Autodesk Inventor part; units mm, degrees
ref_plane "YZ Plane" through (0, 0, 0) normal (1, 0, 0) x (0, 1, 0)
ref_plane "XZ Plane" through (0, 0, 0) normal (0, 1, 0) x (-1, 0, 0)
ref_plane "XY Plane" through (0, 0, 0) normal (0, 0, 1) x (1, 0, 0)
sketch "Sketch1" plane through (0, 0, 0) normal (0, 0, 1) x (1, 0, 0)
  circle A0 centre (0, 0) radius 6.35
  dimension "d0" = 12.7
extrude "Extrusion1" add sketch "Sketch1" along normal blind 203.2
sketch "Sketch4" plane through (0, 0, 0) normal (0, 1, 0) x (-1, 0, 0)
  line L0 (0, 0) -> (0, 1.524)
  line L1 (6.35, 203.2) -> (-6.35, 203.2)
  line L2 (0, 203.2) -> (0, 201.676)
  circle A0 centre (0, 201.676) radius 1.27
  circle A1 centre (0, 1.524) radius 1.27
  dimension "d13" = 1.524
  dimension "d15" = 1.524
  dimension "d16" = 2.54
  dimension "d19" = 2.54
extrude "Extrusion4" cut sketch "Sketch4" along normal mid plane 15.24
sketch "Sketch5" plane through (0, 0, 0) normal (0, 1, 0) x (-1, 0, 0)
  line L0 (0, 1.524) -> (-1.27, 1.524)
  line L1 (-6.35, 0) -> (6.35, 0)
  line L2 (-1.27, 0) -> (1.27, 0)
  line L3 (1.27, 1.524) -> (0, 1.524)
  line L4 (1.27, 1.524) -> (6.35, 1.524)
  line L5 (6.35, 0) -> (6.35, 203.2)
  line L6 (6.35, 1.524) -> (-6.35, 1.524)
  line L7 (-6.35, 1.524) -> (-6.35, 0)
  line L8 (-6.35, 0) -> (6.35, 0)
  line L9 (6.35, 0) -> (6.35, 1.524)
  line L10 (6.35, 203.2) -> (-6.35, 203.2)
  line L11 (-6.35, 203.2) -> (6.35, 203.2)
  line L12 (6.35, 203.2) -> (6.35, 201.676)
  line L13 (6.35, 201.676) -> (-6.35, 201.676)
  line L14 (-6.35, 201.676) -> (-6.35, 203.2)
  point P0 (0, 0)
  dimension "d20" = 1.524
  dimension "d21" = 1.27
  dimension "d26" = 12.7
  dimension "d27" = 1.524
extrude "Extrusion6" cut sketch "Sketch5" along normal mid plane 25.4
sketch "Sketch7" plane through (0, 0, 0) normal (1, 0, 0) x (0, 1, 0)
  line L0 (0, 0) -> (0, 50.8)
  circle A0 centre (0, 50.8) radius 1.27
  line L1 (0, 50.8) -> (0, 101.6)
  circle A1 centre (0, 101.6) radius 1.27
  line L2 (0, 101.6) -> (0, 152.4)
  circle A2 centre (0, 152.4) radius 1.27
  dimension "d42" = 50.8
  dimension "d43" = 2.54
  dimension "d44" = 50.8
  dimension "d45" = 2.54
  dimension "d46" = 50.8
  dimension "d47" = 2.54
extrude "Extrusion8" cut sketch "Sketch7" along normal mid plane 25.4
properties part number "Straw"
Can you work these out from the model? Positions are in its coordinate system, mm. Give positions to 0.01 mm unless a question says otherwise; leave off trailing zeros. Write each loop counter-clockwise with the first axis right and the second up, starting at its lowest first coordinate (ties: lowest second). Pieces come first, ordered by that corner, then holes. Notation, with made-up numbers: (77, 59.5) -> (97, 59.5) arc R16 ccw to (97, 74.5) -> close; hole circle Ø6 at (31, 3). An arc over 180 degrees is marked (long way). One line per item, written item: value.
Q1. For P1, Ø1.5, axis at y = 0, z = 152.4, coming from the +X side; P2, Ø5, axis at x = 4, z = 128.5, coming from the +Y side; P3, Ø4, axis at y = -2.5, z = 62.5, coming from the +X side, each with a flat end and sliding along its axis, tell me the tip position at first contact or that it passes through.
Results found:
P1: passes through
P2: stops at y = 6.17
P3: stops at x = 6.33
Q2. Please list where these lines run through material, in increasing order: line 1 (Z direction, x = 4.25, y = 0); line 2 (Z direction, x = 0, y = 0); line 3 (Y direction, x = 1.75, z = 152.4). Write a range as [from, to].
Results found:
line 1: z = [1.52, 49.53], [52.07, 100.33], [102.87, 151.13], [153.67, 201.68]
line 2: z = [2.79, 49.53], [52.07, 100.33], [102.87, 151.13], [153.67, 200.41]
line 3: y = [-6.1, -1.27], [1.27, 6.1]
Q3. Imagine slicing it at C-C on z = 126. Please give me the cut outline in (x, y).
Results found:
outline: circle Ø12.7 at (0, 0)
Q4. Imagine slicing it at B-B on y = 3.5. Please give me the cut outline in (x, z).
Results found:
outline: (-5.3, 1.52) -> (-1.27, 1.52) arc R1.27 cw to (1.27, 1.52) -> (5.3, 1.52) -> (5.3, 201.68) -> (1.27, 201.68) arc R1.27 cw to (-1.27, 201.68) -> (-5.3, 201.68) -> close
Q5. Imagine slicing it at A-A on x = 3.75. Please give me the cut outline in (y, z), and give its area (3 significant figures).
Results found:
outline: (-5.12, 1.52) -> (5.12, 1.52) -> (5.12, 201.68) -> (-5.12, 201.68) -> close; hole circle Ø2.54 at (0, 50.8); hole circle Ø2.54 at (0, 101.6); hole circle Ø2.54 at (0, 152.4)
area: 2,040 mm^2
